```python
from build123d import *

# Parameters (mm, degrees)
F1_DEPTH  = 8
F3_DEPTH  = 18
F5_DEPTH  = 8
F6_R      = 10
F7_DEPTH  = 1
F9_D      = 3.2
F9_DEPTH  = 8
F9_TIP    = 0.9613769904
F10_R     = 2.5
F11_DEPTH = 15


with BuildPart() as f1:
    # F0 (on Front) → F1 (new body)
    with BuildSketch(Plane.XZ):
        Polygon((-21.15, -17.15), (-17.15, -21.15), (17.15, -21.15), (21.15, -17.15), (21.15, 17.15), (17.15, 21.15), (-17.15, 21.15), (-21.15, 17.15), align=None)
    extrude(amount=F1_DEPTH)

    # F2 (on face) → F3 (join)
    with BuildSketch(Plane.XZ.offset(8)):
        Polygon((-21.15, 15.15), (-21.15, -15.15), (-15.15, -21.15), (15.15, -21.15), (21.15, -15.15), (21.15, 15.15), (15.15, 21.15), (-15.15, 21.15), align=None)
    extrude(amount=F3_DEPTH)

    # F4 (on face) → F5 (join)
    with BuildSketch(Plane.XZ.offset(26)):
        Polygon((-21.15, 17.15), (-21.15, -17.15), (-17.15, -21.15), (17.15, -21.15), (21.15, -17.15), (21.15, 17.15), (17.15, 21.15), (-17.15, 21.15), align=None)
    extrude(amount=F5_DEPTH)

    # F6 (on face) → F7 (join)
    with BuildSketch(Plane.XZ.offset(34)):
        Circle(F6_R)
    extrude(amount=F7_DEPTH)

    # F9
    with Locations(Plane.XZ.offset(34)):
        with Locations((-15.5, 15.5), (15.5, 15.5), (15.5, -15.5), (-15.5, -15.5)):
            Hole(F9_D / 2, depth=F9_DEPTH)
            with Locations((0, 0, -(F9_DEPTH + F9_TIP / 2))):  # 118° drill point
                Cone(0, F9_D / 2, F9_TIP, mode=Mode.SUBTRACT)

    # F10 (on face) → F11 (join)
    with BuildSketch(Plane.XZ.offset(35)):
        Circle(F10_R)
    extrude(amount=F11_DEPTH)


solid = f1.part
```
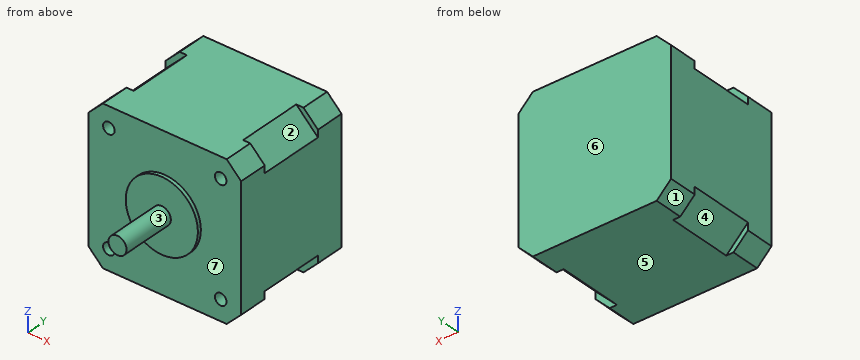
Check sheet for the modelled part. Datum: model origin and axes. Units: mm. Face numbers are marked on the shaded views. A direction names the side the tool comes from. Round coordinates to 2 decimals unless told otherwise and drop trailing zeros. Loops run counter-clockwise (first coordinate to the right, second up) from the corner with the lowest first, then second, coordinate; pieces in that order, holes last. Notation, with made-up numbers: (60.5, -33.75) - (91.5, -33.75) arc R26 ccw to (91.5, -17.75) - close; hole circle Ø10 at (87, 58.5). An arc over 180 degrees is marked (long way). Write item = value, one per line. Start each with the question number.
Q1. Depth check by flat-ended pin: P1, Ø1, axis at x = -15.5, y = -24.5, coming from the +Z side; P2, Ø5, axis at x = 16.5, z = -19.5, coming from the -Y side; P3, Ø2.5, axis at x = 15.5, z = -15.5, coming from the -Y side. Enter the tip coordinate at first touch or a pass-through.
Q2. Access from +Z, -Z, +X, -X, +Y, -Y to the whole of each face (thin tool, end or side, straight path). Record for the marked faces 1, 2 and 3.
Q3. Section check D-D (x = 0). Record the boundary of the cut face in (y, z), plus the area to 3 significant figures.
Q4. Section check B-B (x = 7). Record the boundary of the cut face in (y, z), plus the area to 3 significant figures.
Q5. Section check A-A (z = 0). Record the boundary of the cut face in (x, y), plus the area to 3 significant figures.
Q6. Thickness scan on L1, parallel to Z at x = 15.5, y = -28.75; L2, parallel to Z at x = -15, y = -31. Record the ranges inside material, lowest first.
Q7. Release check for a two-part mould opening along Y. For the marked faces 4, 5, 6 and 7 record: pulls with the +Y half, pulls with the -Y half, needs draft (parallel to the pull), parting line crosses it, or undercut.
Q8. Section check C-C (y = -18). Record the boundary of the cut face in (x, z).
Derived:
q1.P1 = 21.15
q1.P2 = -34
q1.P3 = -25.79
q2.face_1 = -Z, -X, +Y, -Y
q2.face_2 = +Z, +X
q2.face_3 = -Y
q3.outline = (-50, -2.5) - (-35, -2.5) - (-35, -10) - (-34, -10) - (-34, -21.15) - (0, -21.15) - (0, 21.15) - (-34, 21.15) - (-34, 10) - (-35, 10) - (-35, 2.5) - (-50, 2.5) - close
q3.area = 1,530 mm^2
q4.outline = (-35, -7.14) - (-34, -7.14) - (-34, -21.15) - (0, -21.15) - (0, 21.15) - (-34, 21.15) - (-34, 7.14) - (-35, 7.14) - close
q4.area = 1,450 mm^2
q5.outline = (-21.15, -34) - (-10, -34) - (-10, -35) - (-2.5, -35) - (-2.5, -50) - (2.5, -50) - (2.5, -35) - (10, -35) - (10, -34) - (21.15, -34) - (21.15, 0) - (-21.15, 0) - close
q5.area = 1,530 mm^2
q6.L1 = -21.15 to -17.1, -13.9 to 13.9, 17.1 to 21.15
q6.L2 = -21.15 to -17.02, -13.98 to 13.98, 17.02 to 21.15
q7.face_4 = undercut
q7.face_5 = needs draft
q7.face_6 = pulls with the +Y half
q7.face_7 = pulls with the -Y half
q8.outline = (-21.15, -15.15) - (-15.15, -21.15) - (15.15, -21.15) - (21.15, -15.15) - (21.15, 15.15) - (15.15, 21.15) - (-15.15, 21.15) - (-21.15, 15.15) - close
